```python
from build123d import *

# Parameters (mm, degrees)
SKETCH1_W            = 90
SKETCH1_H            = 100
BOSS_EXTRUDE1_DEPTH  = 3
SKETCH2_R            = 6.25
CUT_EXTRUDE1_DEPTH   = 3
LPATTERN1_COUNT      = 3
LPATTERN1_PITCH      = 25
LPATTERN1_COUNT_DIR2 = 2
LPATTERN1_PITCH_DIR2 = 25
SKETCH3_R            = 12
CUT_EXTRUDE2_DEPTH   = 3
M5_CLEARANCE_HOLE1_D = 5.3
FILLET1_R            = 3


with BuildPart() as part:
    # Sketch1 → Boss-Extrude1 (new body)
    with BuildSketch(Plane(origin=(0, 0, 0), x_dir=(1, 0, 0), z_dir=(0, 1, 0))):
        with Locations((45, 50)):
            Rectangle(SKETCH1_W, SKETCH1_H)
    extrude(amount=BOSS_EXTRUDE1_DEPTH)

    # Sketch2 → Cut-Extrude1 (cut)
    with BuildSketch(Plane(origin=(0, 3, 0), x_dir=(1, 0, 0), z_dir=(0, 1, 0))):
        with Locations(Location((20, 20, 0), (0, 0, 270))):
            Circle(SKETCH2_R)
    cut_extrude1 = extrude(amount=-CUT_EXTRUDE1_DEPTH, mode=Mode.SUBTRACT)

    # LPattern1: Cut-Extrude1 3 × 2
    with Locations(*[(i * LPATTERN1_PITCH, 0, -j * LPATTERN1_PITCH_DIR2) for i in range(LPATTERN1_COUNT) for j in range(LPATTERN1_COUNT_DIR2) if (i, j) != (0, 0)]):
        add(cut_extrude1, mode=Mode.SUBTRACT)

    # Sketch3 → Cut-Extrude2 (cut)
    with BuildSketch(Plane(origin=(0, 3, 0), x_dir=(1, 0, 0), z_dir=(0, 1, 0))):
        with Locations(Location((25, 75.625, 0), (0, 0, 270))):
            Circle(SKETCH3_R)
        with Locations(Location((65, 75.625, 0), (0, 0, 270))):
            Circle(SKETCH3_R)
    extrude(amount=-CUT_EXTRUDE2_DEPTH, mode=Mode.SUBTRACT)

    # M5 Clearance Hole1 (through all)
    with Locations(Plane(origin=(0, 3, 0), x_dir=(1, 0, 0), z_dir=(0, 1, 0))):
        with Locations((5, 95), (5, 5), (85, 5), (85, 95)):
            Hole(M5_CLEARANCE_HOLE1_D / 2)

    # Fillet1
    fillet1_edges = [part.edges().sort_by_distance(p)[0] for p in [
        (0, 1.5, -100),
        (90, 1.5, -100),
        (90, 1.5, 0),
        (0, 1.5, 0),
    ]]
    fillet(fillet1_edges, radius=FILLET1_R)


solid = part.part
```
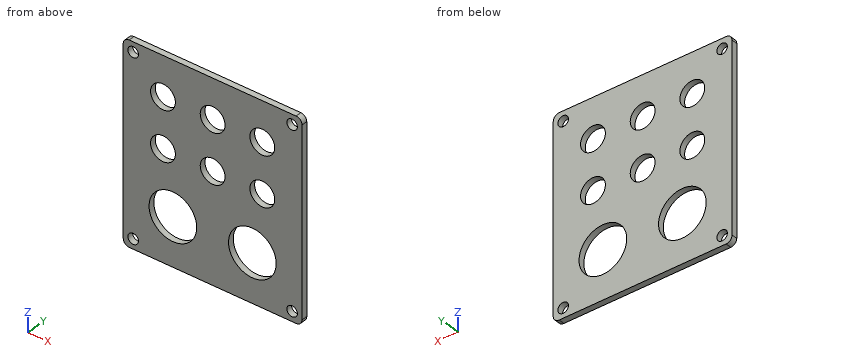
Geometry: final body of the model. Coordinates: model frame, mm. Round coordinates to 2 decimals unless told otherwise and drop trailing zeros. Order: outer loops, then holes, each group sorted by start corner. A loop starts at its lowest first (then second) coordinate and runs counter-clockwise, first axis right, second up. Notation, with made-up numbers: (28, 64.5) - (57, 64.5) arc R14 ccw to (57, 81.5) - close; hole circle Ø4 at (15.5, 64). An arc over 180 degrees is marked (long way). Write item = value, one per line. Start each with the question number.
Q1. Cut plane A-A on z = -20. Return the cut outline in (x, y).
Q2. Ray query, line 1 (X direction, y = 1.65, z = -95); line 2 (Z direction, x = 5, y = 2.1); line 3 (X direction, y = 2.6, z = -22). Return the intervals inside material, ascending. Write a range as from..to.
Q3. Cut plane B-B on x = 65. Return the cut outline in (y, z) (3 decimals).
Q4. Cut plane D-D on y = 2.2. Give the number of separate pieces and of enclosed holes in the cut face, and give its area (3 significant figures).
Q5. Cut plane C-C on x = 45. Return the cut outline in (y, z), and give its area (3 significant figures).
Outcome:
q1.outline = (0, 0) - (13.75, 0) - (13.75, 3) - (0, 3) - close; (26.25, 0) - (38.75, 0) - (38.75, 3) - (26.25, 3) - close; (51.25, 0) - (63.75, 0) - (63.75, 3) - (51.25, 3) - close; (76.25, 0) - (90, 0) - (90, 3) - (76.25, 3) - close
q2.line_1 = 0..2.35, 7.65..82.35, 87.65..90
q2.line_2 = -100..-97.65, -92.35..-7.65, -2.35..0
q2.line_3 = 0..14.08, 25.92..39.08, 50.92..64.08, 75.92..90
q3.outline = (0, -100) - (3, -100) - (3, -87.625) - (0, -87.625) - close; (0, -63.625) - (3, -63.625) - (3, -48.75) - (0, -48.75) - close; (0, -41.25) - (3, -41.25) - (3, -23.75) - (0, -23.75) - close; (0, -16.25) - (3, -16.25) - (3, 0) - (0, 0) - close
q4.separate_pieces = 1
q4.enclosed_holes = 12
q4.area = 7,260 mm^2
q5.outline = (0, -100) - (3, -100) - (3, -51.25) - (0, -51.25) - close; (0, -38.75) - (3, -38.75) - (3, -26.25) - (0, -26.25) - close; (0, -13.75) - (3, -13.75) - (3, 0) - (0, 0) - close
q5.area = 225 mm^2
